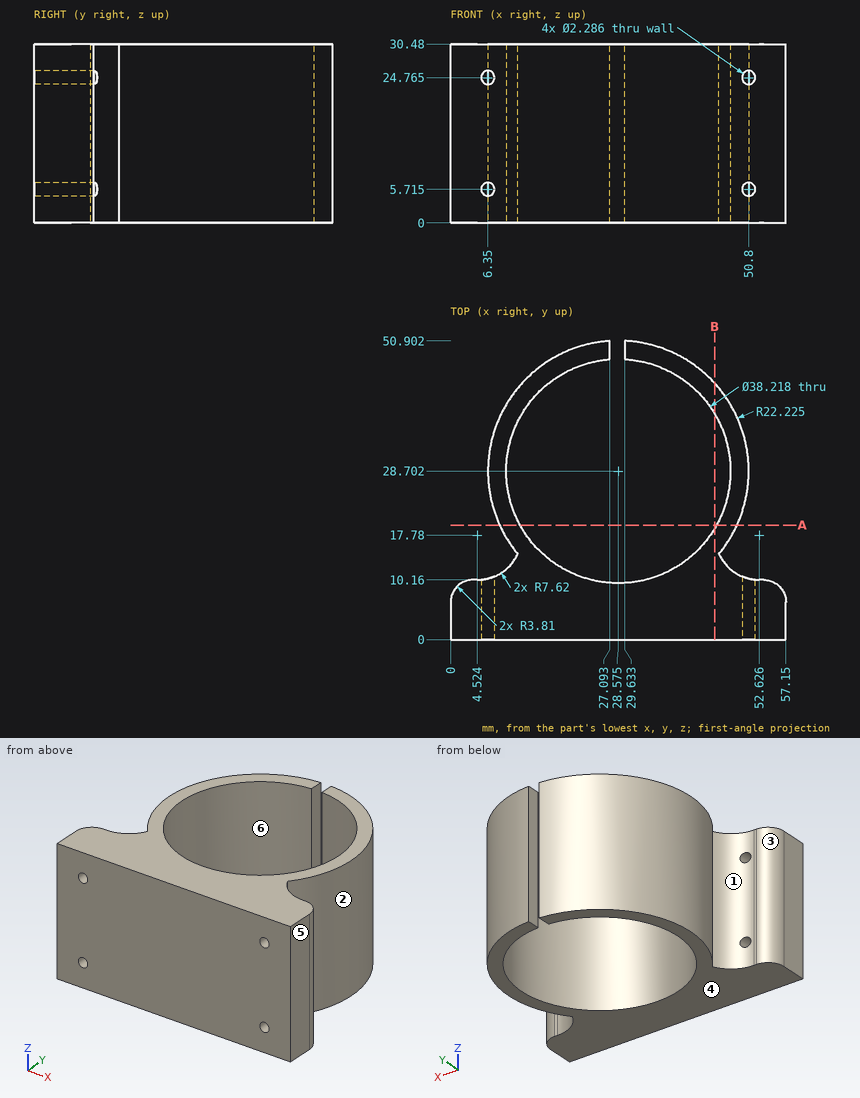
Input: dimensioned drawing with shaded views. Units: mm. Origin: part minimum x, y, z. A direction names the side the tool comes from. Round coordinates to 2 decimals unless told otherwise and drop trailing zeros. Loops run counter-clockwise (first coordinate to the right, second up) from the corner with the lowest first, then second, coordinate; pieces in that order, holes last. Notation, with made-up numbers: M 52,32.5 L 71,32.5 A8 ccw 71,41.5 Z; hole C 56,-16 d10. An arc over 180 degrees is marked long. Return JSON: item names as keys, results as strings. Group by question number.
1. Reachability of the marked faces 1 and 2 from +Z, -Z, +X, -X, +Y, -Y: full face, straight path, thin tool, end or side. Return the list, or none.
2. Material intervals for line 1 along Z through (x, y) = (6.35, 7.75); line 2 along Y through (x, z) = (11, 15.5) (1 decimal); line 3 along Y through (x, z) = (24, 16) (1 decimal), sorted ascending. Write a range as from..to.
3. Section query B-B on x = 45. Output: boundary loops of the cut face in (y, z), and give its area (3 significant figures).
4. Section query A-A on y = 19.5. Output: boundary loops of the cut face in (x, z) (1 decimal).
5. Pin query (flat end, axial travel): pin 1 (2 mm diameter, centred on x = 48, z = 25, fed in from +Y); pin 2 (1.6 mm diameter, centred on y = 49, z = 16.5, fed in from +X); pin 3 (3 mm diameter, centred on y = 24, z = 8.5, fed in from +X). Return the tip coordinate at first contact, or that it passes through.
6. Mould query, pull axis X, two halves, no side actions, for the marked faces 3, 4, 5 and 6. Classes: released by +X, released by -X, zero draft, split by the parting line, or undercut.
Checks:
{
 "1": {"face 1": "+Z, -Z, -X", "face 2": "+Z, -Z, +X"},
 "2": {"line 1": "z = 0..4.57, 6.86..23.62, 25.91..30.48", "line 2": "y = 0..13.8, 15.1..21.2, 36.2..42.3", "line 3": "y = 0..10.1, 47.3..50.5"},
 "3": {"outline": "M 0,0 L 18.94,0 L 18.94,30.48 L 0,30.48 Z; M 38.47,0 L 43.67,0 L 43.67,30.48 L 38.47,30.48 Z", "area": "736 mm²"},
 "4": {"outline": "M 8.3,0 L 11.8,0 L 11.8,30.5 L 8.3,30.5 Z; M 45.3,0 L 48.8,0 L 48.8,30.5 L 45.3,30.5 Z"},
 "5": {"pin 1": "stops at y = 41.13", "pin 2": "stops at x = 39.24", "pin 3": "stops at x = 50.57"},
 "6": {"face 3": "released by -X", "face 4": "zero draft", "face 5": "released by +X", "face 6": "undercut"}
}
